Geometry: final body of the model. Coordinates: model frame, mm. Face numbers are marked on the shaded views. A direction names the side the tool comes from. Give positions to 0.01 mm unless a question says otherwise; leave off trailing zeros. Write each loop counter-clockwise with the first axis right and the second up, starting at its lowest first coordinate (ties: lowest second). Pieces come first, ordered by that corner, then holes. Notation, with made-up numbers: (-2.5, 5.25) -> (15.5, 5.25) arc R33 ccw to (15.5, 40.25) -> close; hole circle Ø4 at (-27, 88). An arc over 180 degrees is marked (long way). Use CSV: the item, a comma, the result in double quotes. Start each with the question number.
1) Set-up query: the marked faces 1, 2 and 3. Return all of +Z, -Z, +X, -X, +Y, -Y with unobstructed straight access to the full face (end or side cutting, diameter ignored); none if empty.
2) Material intervals for line 1 (Z direction, x = 7.25, y = -8.75); line 2 (X direction, y = -11, z = -134.5); line 3 (X direction, y = -2.5, z = -173.5), sorted ascending. Write a range as [from, to].
3) Section C-C (z = -121). Output: boundary loops of the cut face in (x, y), plus the area to 3 significant figures.
4) Contact query for flat-ended pins moving along their axis: P1, Ø10, axis at y = -6, z = -59, coming from the -X side; P2, Ø1, axis at x = 12, z = -147, coming from the +Y side; P3, Ø1, axis at x = 9.5, z = -27, coming from the +Y side. Output: stop coordinate, or through.
5) Section D-D (z = -12.5). Output: boundary loops of the cut face in (x, y).
6) Section A-A (y = 0). Output: boundary loops of the cut face in (x, z).
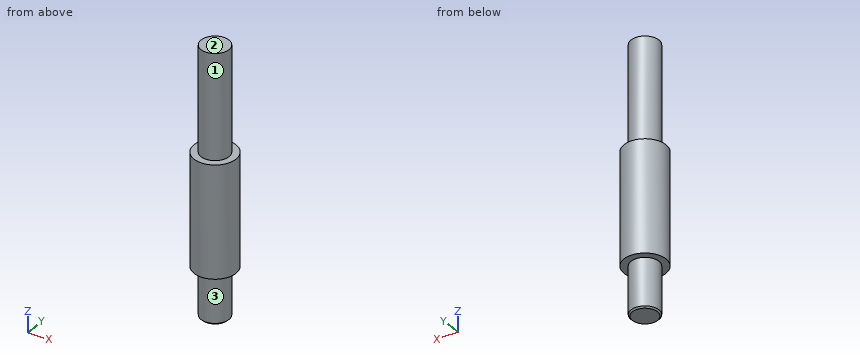
```python
from build123d import *

# Parameters (mm, degrees)
SKETCH1_R           = 10.01
BOSS_EXTRUDE1_DEPTH = 75
SKETCH2_R           = 15
BOSS_EXTRUDE2_DEPTH = 80
SKETCH3_R           = 10.01
BOSS_EXTRUDE3_DEPTH = 35
CHAMFER1_SIZE       = 1


with BuildPart() as part:
    # Sketch1 → Boss-Extrude1 (new body)
    with BuildSketch(Plane.XY):
        Circle(SKETCH1_R)
    extrude(amount=-BOSS_EXTRUDE1_DEPTH)

    # Sketch2 → Boss-Extrude2 (add)
    with BuildSketch(Plane(origin=(0, 0, -75), x_dir=(-1, 0, 0), z_dir=(0, 0, -1))):
        Circle(SKETCH2_R)
    extrude(amount=BOSS_EXTRUDE2_DEPTH)

    # Sketch3 → Boss-Extrude3 (add)
    with BuildSketch(Plane(origin=(0, 0, -155), x_dir=(-1, 0, 0), z_dir=(0, 0, -1))):
        Circle(SKETCH3_R)
    extrude(amount=BOSS_EXTRUDE3_DEPTH)

    # Chamfer1
    chamfer1_edges = [part.edges().sort_by_distance(p)[0] for p in [
        (10.01, 0, -190),
    ]]
    chamfer(chamfer1_edges, length=CHAMFER1_SIZE)


solid = part.part
```
Answers follow:
1,face 1,"+Z"
1,face 2,"+Z, +X, -X, +Y, -Y"
1,face 3,"-Z"
2,line 1,"z = [-155, -75]"
2,line 2,"x = [-10.2, 10.2]"
2,line 3,"x = [-9.69, 9.69]"
3,outline,"circle Ø30 at (0, 0)"
3,area,"707 mm^2"
4,P1,"stops at x = -9.96"
4,P2,"stops at y = 9.63"
4,P3,"stops at y = 4.38"
5,outline,"circle Ø20.02 at (0, 0)"
6,outline,"(-15, -155) -> (-10.01, -155) -> (-10.01, -189) -> (-9.01, -190) -> (9.01, -190) -> (10.01, -189) -> (10.01, -155) -> (15, -155) -> (15, -75) -> (10.01, -75) -> (10.01, 0) -> (-10.01, 0) -> (-10.01, -75) -> (-15, -75) -> close"
